Answer from the drawing. Dimensions are ordinates in mm from the lowest x, y and z of the part. A direction names the side the tool comes from. Coordinates: 2 decimals unless noted, no trailing zeros. Loops run counter-clockwise (first coordinate to the right, second up) from the corner with the lowest first, then second, coordinate; pieces in that order, holes last.
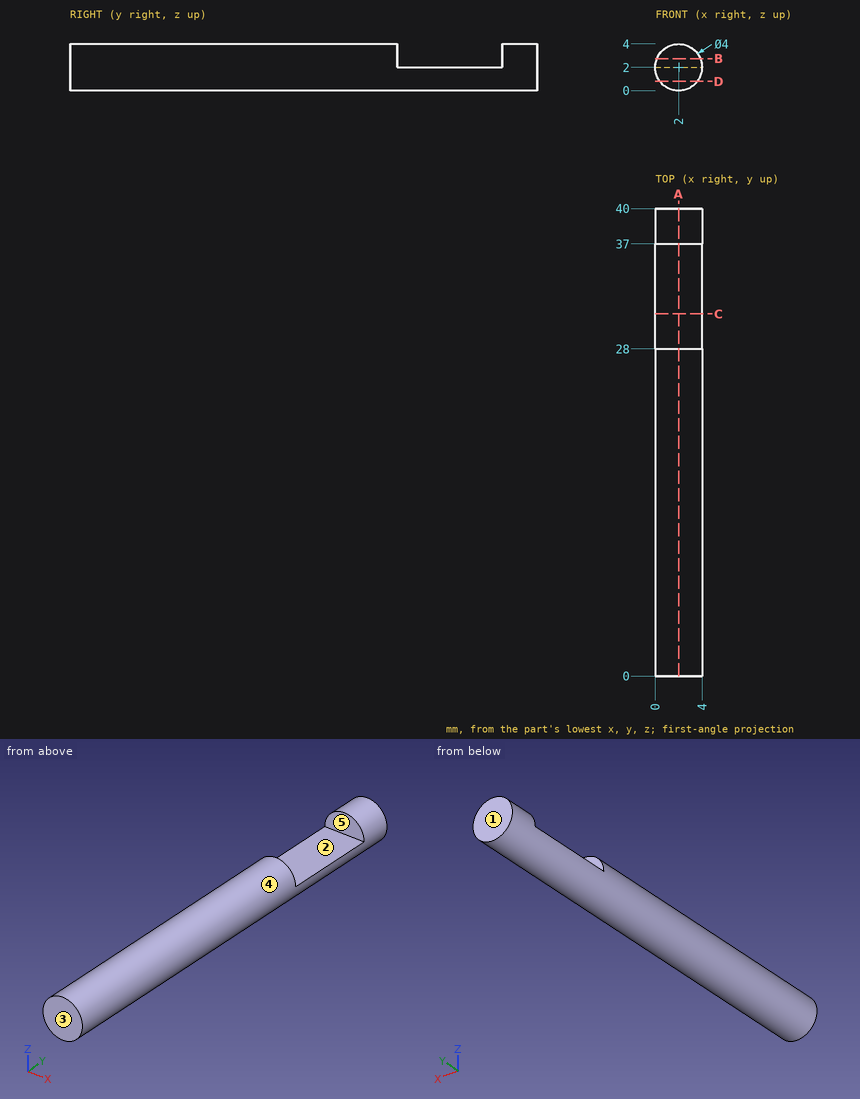
Item 1: A cutting plane is placed at A-A on x = 2. Determine the outline of the cut face in (y, z).
Numbers:
outline: (0, 0) - (40, 0) - (40, 4) - (37, 4) - (37, 2) - (28, 2) - (28, 4) - (0, 4) - close
Item 2: A cutting plane is placed at B-B on z = 2.75. Determine the outline of the cut face in (x, y).
Numbers:
outline: (0.15, 0) - (3.85, 0) - (3.85, 28) - (0.15, 28) - close; (0.15, 37) - (3.85, 37) - (3.85, 40) - (0.15, 40) - close
Item 3: Determine the mould class of the marked faces 3, 4 and 5 for opening direction Y: released by +Y, released by -Y, zero draft, split by the parting line, or undercut.
Numbers:
face 3: released by -Y
face 4: zero draft
face 5: undercut
Item 4: A cutting plane is placed at C-C on y = 31. Determine the outline of the cut face in (x, z), then the cut area to 3 significant figures.
Numbers:
outline: (0, 2) arc R2 ccw to (4, 2) - close
area: 6.28 mm2
Item 5: Find the intervals of material crossed by line 1 along Y through (x, z) = (3.8, 2.7); line 2 along Z through (x, y) = (1.85, 9); line 3 along X through (y, z) = (25.5, 1.7), in increasing order.
Numbers:
line 1: y = 0 to 28, 37 to 40
line 2: z = 0.01 to 3.99
line 3: x = 0.02 to 3.98
Item 6: A cutting plane is placed at D-D on z = 0.8. Determine the outline of the cut face in (x, y).
Numbers:
outline: (0.4, 0) - (3.6, 0) - (3.6, 40) - (0.4, 40) - close
Item 7: Which of the six approach directions +Z, -Z, +X, -X, +Y, -Y give full straight-line access (tool end or side, diameter ignored) to the marked faces 1 and 2?
Numbers:
face 1: +Z, -Z, +X, -X, +Y
face 2: +Z, +X, -X
Item 8: Given pin 1 (1 mm diameter, centred on y = 30.5, z = 0.5, fed in from -X), flat-ended and moving along its own axis, determine where the tip first touches the part or whether it passes through.
Numbers:
pin 1: stops at x = 0.27
